Part model, mm, in its own coordinate system. A direction names the side the tool comes from. Coordinates: 2 decimals unless noted, no trailing zeros. Write each loop counter-clockwise with the first axis right and the second up, starting at its lowest first coordinate (ties: lowest second). Pieces come first, ordered by that corner, then holes. Notation, with made-up numbers: (69.25, 34.25) -> (104.25, 34.25) arc R15 ccw to (104.25, 40.25) -> close; hole circle Ø3 at (52, 39). An arc over 180 degrees is marked (long way). Write item = value, one per line.
from build123d import *

# Parameters (mm, degrees)
F1_DEPTH = 300


with BuildPart() as f1:
    # F0 (on Top) → F1 (new body)
    with BuildSketch(Plane.XY):
        Polygon((0, 7), (0, 0), (7, 0), (7, 5.5), (13, 5.5), (13, 0), (20, 0), (20, 7), (14.5, 7), (14.5, 13), (20, 13), (20, 20), (13, 20), (13, 14.5), (7, 14.5), (7, 20), (0, 20), (0, 13), (5.5, 13), (5.5, 7), align=None)
        Polygon((-7, 0), (0, 0), (0, 7), (-5.5, 7), (-5.5, 13), (0, 13), (0, 20), (-7, 20), (-7, 14.5), (-13, 14.5), (-13, 20), (-20, 20), (-20, 13), (-14.5, 13), (-14.5, 7), (-20, 7), (-20, 0), (-13, 0), (-13, 5.5), (-7, 5.5), align=None)
        Polygon((0, -7), (0, 0), (-7, 0), (-7, -5.5), (-13, -5.5), (-13, 0), (-20, 0), (-20, -7), (-14.5, -7), (-14.5, -13), (-20, -13), (-20, -20), (-13, -20), (-13, -14.5), (-7, -14.5), (-7, -20), (0, -20), (0, -13), (-5.5, -13), (-5.5, -7), align=None)
        Polygon((7, 0), (0, 0), (0, -7), (5.5, -7), (5.5, -13), (0, -13), (0, -20), (7, -20), (7, -14.5), (13, -14.5), (13, -20), (20, -20), (20, -13), (14.5, -13), (14.5, -7), (20, -7), (20, 0), (13, 0), (13, -5.5), (7, -5.5), align=None)
    extrude(amount=F1_DEPTH)


solid = f1.part
Q1. Saw through at C-C on y = -10. Give the cut face in (x, z).
Model answer:
outline = (-14.5, 0) -> (-5.5, 0) -> (-5.5, 300) -> (-14.5, 300) -> close; (5.5, 0) -> (14.5, 0) -> (14.5, 300) -> (5.5, 300) -> close
Q2. Which spindle directions (+Z, -Z, +X, -X, +Y, -Y) get a long thin tool onto all of the face, cutting with end or side? Do faces 1 (the face through (-10, 14.5, 148)), 2 (the face through (-7, -17, 148)), 3 (the face through (-17, -13, 148)), 4 (the face through (-10, -5.5, 148)). Say none if no direction does.
Model answer:
face_1 = +Z, -Z, +Y
face_2 = +Z, -Z, -Y
face_3 = +Z, -Z, -X
face_4 = +Z, -Z
Q3. Saw through at A-A on y = 1.5. Give the cut face in (x, z).
Model answer:
outline = (-20, 0) -> (-13, 0) -> (-13, 300) -> (-20, 300) -> close; (-7, 0) -> (7, 0) -> (7, 300) -> (-7, 300) -> close; (13, 0) -> (20, 0) -> (20, 300) -> (13, 300) -> close
Q4. Pin check, flat tips, straight feed: pin 1 (2 mm diameter, centred on y = -10.5, z = 261, fed in from -X); pin 2 (2 mm diameter, centred on x = 10.5, z = 85, fed in from +Y); pin 3 (1.8 mm diameter, centred on y = 11.5, z = 106.5, fed in from +X). Stop position of each tip, or through.
Model answer:
pin_1 = -14.5
pin_2 = 14.5
pin_3 = 14.5
Q5. Probe line 1 (X direction, y = -4.5, z = 282.5); line 2 (Y direction, x = 7.5, z = 117). List the from-to ranges inside material, lowest first. Write a range as from..to.
Model answer:
line_1 = -20..-13, -7..7, 13..20
line_2 = -14.5..-5.5, 5.5..14.5
Q6. Mould opens along X. For faces 5 (the face through (10, 5.5, 148)), 6 (the face through (20, 16, 148)), 7 (the face through (-20, 17, 148)) say: released by +X, released by -X, zero draft, split by the parting line, or undercut.
Model answer:
face_5 = undercut
face_6 = released by +X
face_7 = released by -X
Q7. Saw through at D-D on z = 168.5. Count the separate pieces of the cut face and the enclosed holes in it, and give its area (3 significant figures).
Model answer:
separate_pieces = 1
enclosed_holes = 4
area = 1,070 mm²
